Here's how the part is built. I have some questions about the finished solid (model axes, mm). A direction names the side the tool comes from. Coordinates: 2 decimals unless noted, no trailing zeros. Loops run counter-clockwise (first coordinate to the right, second up) from the corner with the lowest first, then second, coordinate; pieces in that order, holes last. Notation, with made-up numbers: (19, -38.75) -> (44, -38.75) arc R14 ccw to (44, -18.75) -> close; hole circle Ø1 at (48.5, -19.5). An arc over 180 degrees is marked (long way). Use CSV: the item, a comma, the result in double quotes. Start each with the question number.
from build123d import *

# Parameters (mm, degrees)
SKETCH1_W           = 50
SKETCH1_H           = 40
BOSS_EXTRUDE1_DEPTH = 10
SKETCH5_W           = 6
SKETCH5_H           = 5
BOSS_EXTRUDE3_DEPTH = 10
SKETCH6_R           = 2
CUT_EXTRUDE1_DEPTH  = 20
SKETCH8_W           = 10
SKETCH8_H           = 40
CUT_EXTRUDE2_DEPTH  = 25
SKETCH9_W           = 10
SKETCH9_H           = 6
SKETCH9_R           = 1.930897171
BOSS_EXTRUDE4_DEPTH = 5
SKETCH10_W          = 10
SKETCH10_H          = 5
CUT_EXTRUDE3_DEPTH  = 15
SKETCH11_W          = 5
SKETCH11_H          = 5
BOSS_EXTRUDE5_DEPTH = 10
SKETCH12_R          = 1.5
CUT_EXTRUDE4_DEPTH  = 10
CUT_EXTRUDE5_DEPTH  = 10
CUT_EXTRUDE6_DEPTH  = 10


with BuildPart() as part:
    # Sketch1 → Boss-Extrude1 (new body)
    with BuildSketch(Plane(origin=(669.84184187, 0, 0), x_dir=(1, 0, 0), z_dir=(0, 0, 1))):
        with Locations((-671.310344828, 437.637931034)):
            Rectangle(SKETCH1_W, SKETCH1_H)
    boss_extrude1 = extrude(amount=BOSS_EXTRUDE1_DEPTH)

    # Sketch5 → Boss-Extrude3 (add)
    with BuildSketch(Plane(origin=(23.531497042, 0, 0), x_dir=(0, 0, -1), z_dir=(1, 0, 0))):
        with Locations((-5, 442.637931034)):
            Rectangle(SKETCH5_W, SKETCH5_H)
        with Locations((-5, 432.637931034)):
            Rectangle(SKETCH5_W, SKETCH5_H)
    extrude(amount=BOSS_EXTRUDE3_DEPTH)

    # Sketch6 → Cut-Extrude1 (cut)
    with BuildSketch(Plane(origin=(669.84184187, 445.137931034, 0), x_dir=(1, 0, 0), z_dir=(0, 1, 0))):
        with Locations(Location((-641.310344828, -5, 0), (0, 0, 180))):
            Circle(SKETCH6_R)
    extrude(amount=-CUT_EXTRUDE1_DEPTH, mode=Mode.SUBTRACT)

    # Sketch8 → Cut-Extrude2 (cut)
    with BuildSketch(Plane.ZY.offset(26.468502958)):
        with Locations((5, 437.637931034)):
            Rectangle(SKETCH8_W, SKETCH8_H)
    extrude(amount=-CUT_EXTRUDE2_DEPTH, mode=Mode.SUBTRACT)

    # Sketch9 → Boss-Extrude4 (add)
    with BuildSketch(Plane(origin=(0, 435.137931034, 0), x_dir=(1, 0, 0), z_dir=(0, 1, 0))):
        with Locations((28.531497042, -5)):
            Rectangle(SKETCH9_W, SKETCH9_H)
        with Locations(Location((28.531497042, -5, 0), (0, 0, 180))):
            Circle(SKETCH9_R, mode=Mode.SUBTRACT)
    extrude(amount=BOSS_EXTRUDE4_DEPTH)

    # Sketch10 → Cut-Extrude3 (cut)
    with BuildSketch(Plane.XY.offset(8)):
        with Locations((28.531497042, 432.637931034)):
            Rectangle(SKETCH10_W, SKETCH10_H)
        with Locations((28.531497042, 442.637931034)):
            Rectangle(SKETCH10_W, SKETCH10_H)
    extrude(amount=-CUT_EXTRUDE3_DEPTH, mode=Mode.SUBTRACT)

    # Mirror1: Boss-Extrude1 across plane
    add(boss_extrude1.mirror(Plane(origin=(-1.468502958, 0, 0), x_dir=(0, 0, 1), z_dir=(1, 0, 0))))

    # Sketch11 → Boss-Extrude5 (add)
    with BuildSketch(Plane(origin=(0, 457.637931034, 0), x_dir=(1, 0, 0), z_dir=(0, 1, 0))):
        with Locations((-1.468502958, -5)):
            Rectangle(SKETCH11_W, SKETCH11_H)
    extrude(amount=BOSS_EXTRUDE5_DEPTH)

    # Sketch12 → Cut-Extrude4 (cut)
    with BuildSketch(Plane(origin=(1.031497042, 0, 0), x_dir=(0, 0, -1), z_dir=(1, 0, 0))):
        with Locations((-5, 462.637931034)):
            Circle(SKETCH12_R)
    extrude(amount=-CUT_EXTRUDE4_DEPTH, mode=Mode.SUBTRACT)

    # Sketch13 → Cut-Extrude5 (cut)
    with BuildSketch(Plane(origin=(1.031497042, 0, 0), x_dir=(0, 0, -1), z_dir=(1, 0, 0))):
        with BuildLine():
            Line((-7.5, 467.637931034), (-7.5, 462.637931034))
            ThreePointArc((-7.5, 462.637931034), (-5, 465.137931034), (-2.5, 462.637931034))
            Line((-2.5, 462.637931034), (-2.5, 467.637931034))
            Line((-2.5, 467.637931034), (-7.5, 467.637931034))
        make_face()
    extrude(amount=-CUT_EXTRUDE5_DEPTH, mode=Mode.SUBTRACT)

    # Sketch14 → Cut-Extrude6 (cut)
    with BuildSketch(Plane(origin=(0, 440.137931034, 0), x_dir=(1, 0, 0), z_dir=(0, 1, 0))):
        with BuildLine():
            Line((33.531497042, -2), (28.531497042, -2))
            ThreePointArc((28.531497042, -2), (30.652817386, -2.878679656), (31.531497042, -5))
            ThreePointArc((31.531497042, -5), (30.652817386, -7.121320344), (28.531497042, -8))
            Line((28.531497042, -8), (33.531497042, -8))
            Line((33.531497042, -8), (33.531497042, -2))
        make_face()
    extrude(amount=-CUT_EXTRUDE6_DEPTH, mode=Mode.SUBTRACT)


solid = part.part
1) Thinking about a two-plate mould opening in X: for faces 5 (the face through (1.031, 460.5, 5)), 6 (the face through (26.69, 437.6, 5.58)), 7 (the face through (-2, 460, 7.5)), which applies, pulls with the +X half, pulls with the -X half, needs draft (parallel to the pull), parting line crosses it, or undercut?
2) Which directions (+Z, -Z, +X, -X, +Y, -Y) give clear straight access to the entire face, cutting with the end or side of a thin tool? Please do faces 1 (the face through (-3.969, 460.5, 5)), 2 (the face through (26, 440.138, 5)), 3 (the face through (26, 438, 8)), 4 (the face through (26, 435.138, 5)).
3) I want a section at C-C, the plane z = 4.25. Please give me the cut outline in (x, y).
4) I want a section at B-B, the plane y = 438. Please give me the cut outline in (x, z).
5) Please list where these lines run through material, in increasing order: L1, parallel to X at y = 454.5, z = 9.75; L2, parallel to Y at x = -1.5, z = 9.75; L3, parallel to Y at x = -1.5, z = 5. Write a range as [from, to].
6) For P1, Ø1.5, axis at y = 451.5, z = 8.5, coming from the +X side; P2, Ø5.5, axis at y = 463, z = 4, coming from the -X side; P3, Ø2, axis at y = 436.5, z = 6.5, coming from the +X side, each with a flat end and sliding along its axis, tell me the tip position at first contact or that it passes through.
7) I want a section at D-D, the plane y = 455. Please give me the cut outline in (x, z), plus the area to 3 significant figures.
8) I want a section at A-A, the plane x = -2. Please give me the cut outline in (y, z), plus the area to 3 significant figures.
Return value:
1,face 5,"pulls with the +X half"
1,face 6,"undercut"
1,face 7,"needs draft"
2,face 1,"+Z, -Z, -X, +Y"
2,face 2,"+Z, -Z, +X, +Y"
2,face 3,"+Z, +X, +Y, -Y"
2,face 4,"+Z, -Z, +X, -Y"
3,outline,"(-26.47, 417.64) -> (23.53, 417.64) -> (23.53, 435.14) -> (26.75, 435.14) -> (26.75, 440.14) -> (23.53, 440.14) -> (23.53, 457.64) -> (1.03, 457.64) -> (1.03, 461.34) -> (-3.97, 461.34) -> (-3.97, 457.64) -> (-26.47, 457.64) -> close; (-3.97, 463.94) -> (1.03, 463.94) -> (1.03, 465.02) -> (-3.97, 465.02) -> close; (30.31, 435.14) -> (31.44, 435.14) -> (31.44, 440.14) -> (30.31, 440.14) -> close"
4,outline,"(-26.47, 0) -> (23.53, 0) -> (23.53, 2) -> (28.53, 2) arc R3 ccw to (28.53, 8) -> (23.53, 8) -> (23.53, 10) -> (-26.47, 10) -> close; hole circle Ø3.86 at (28.53, 5)"
5,L1,"x = [-26.47, 23.53]"
5,L2,"y = [417.64, 457.64]"
5,L3,"y = [417.64, 461.14], [464.14, 465.14]"
6,P1,"stops at x = 23.53"
6,P2,"stops at x = -3.97"
6,P3,"stops at x = 31.49"
7,outline,"(-26.47, 0) -> (23.53, 0) -> (23.53, 10) -> (-26.47, 10) -> close"
7,area,"500 mm²"
8,outline,"(417.64, 0) -> (457.64, 0) -> (457.64, 2.5) -> (462.64, 2.5) arc R2.5 ccw to (462.64, 7.5) -> (457.64, 7.5) -> (457.64, 10) -> (417.64, 10) -> close; hole circle Ø3 at (462.64, 5)"
8,area,"428 mm²"
